from build123d import *

# Parameters (mm, degrees)
SKETCH1_W           = 270
SKETCH1_H           = 180
BOSS_EXTRUDE1_DEPTH = 6
SKETCH2_R           = 1.6
CUT_EXTRUDE1_DEPTH  = 7
SKETCH3_R           = 1.6
CUT_EXTRUDE2_DEPTH  = 10
SKETCH4_R           = 1.6
SKETCH4_R_2         = 1.5
CUT_EXTRUDE3_DEPTH  = 7
SKETCH5_R           = 1.6
CUT_EXTRUDE4_DEPTH  = 10
SKETCH6_R           = 2.1
CUT_EXTRUDE5_DEPTH  = 10


with BuildPart() as part:
    # Sketch1 → Boss-Extrude1 (new body)
    with BuildSketch(Plane(origin=(0, 0, 0), x_dir=(1, 0, 0), z_dir=(0, 1, 0))):
        Rectangle(SKETCH1_W, SKETCH1_H)
    extrude(amount=BOSS_EXTRUDE1_DEPTH)

    # Sketch2 → Cut-Extrude1 (cut, through all)
    with BuildSketch(Plane.XZ):
        with Locations((-122, 81.5)):
            Circle(SKETCH2_R)
        with Locations((-100.000000181, 81.5)):
            Circle(SKETCH2_R)
        with Locations((-122, 6.500000003)):
            Circle(SKETCH2_R)
        with Locations((-100.000000181, 6.500000003)):
            Circle(SKETCH2_R)
        with Locations((-122, 21.000003407)):
            Circle(SKETCH2_R)
        with Locations((-122, 49.000003407)):
            Circle(SKETCH2_R)
    extrude(amount=-CUT_EXTRUDE1_DEPTH, mode=Mode.SUBTRACT)

    # Sketch3 → Cut-Extrude2 (cut)
    with BuildSketch(Plane.XZ):
        with Locations((-40, -39)):
            Circle(SKETCH3_R)
        with Locations((-40, -75)):
            Circle(SKETCH3_R)
        with Locations((-4, -75)):
            Circle(SKETCH3_R)
        with Locations((-4, -39)):
            Circle(SKETCH3_R)
        with BuildLine():
            Line((-29.38, -15.458502607), (-29.38, -5.458502607))
            ThreePointArc((-29.38, -5.458502607), (-27.38, -3.458502607), (-25.38, -5.458502607))
            Line((-25.38, -5.458502607), (-25.38, -15.458502607))
            ThreePointArc((-25.38, -15.458502607), (-27.38, -17.458502607), (-29.38, -15.458502607))
        make_face()
        with BuildLine():
            Line((-14.63, -15.458502607), (-14.63, -5.458502607))
            ThreePointArc((-14.63, -5.458502607), (-16.63, -3.458502607), (-18.63, -5.458502607))
            Line((-18.63, -5.458502607), (-18.63, -15.458502607))
            ThreePointArc((-18.63, -15.458502607), (-16.63, -17.458502607), (-14.63, -15.458502607))
        make_face()
        with BuildLine():
            Line((-29.38, 24.541497393), (-29.38, 34.541497393))
            ThreePointArc((-29.38, 34.541497393), (-27.38, 36.541497393), (-25.38, 34.541497393))
            Line((-25.38, 34.541497393), (-25.38, 24.541497393))
            ThreePointArc((-25.38, 24.541497393), (-27.38, 22.541497393), (-29.38, 24.541497393))
        make_face()
        with BuildLine():
            Line((-14.63, 24.541497393), (-14.63, 34.541497393))
            ThreePointArc((-14.63, 34.541497393), (-16.63, 36.541497393), (-18.63, 34.541497393))
            Line((-18.63, 34.541497393), (-18.63, 24.541497393))
            ThreePointArc((-18.63, 24.541497393), (-16.63, 22.541497393), (-14.63, 24.541497393))
        make_face()
    extrude(amount=-CUT_EXTRUDE2_DEPTH, mode=Mode.SUBTRACT)

    # Sketch4 → Cut-Extrude3 (cut, through all)
    with BuildSketch(Plane(origin=(0, 6, 0), x_dir=(1, 0, 0), z_dir=(0, 1, 0))):
        with Locations((19.999964, -14)):
            Circle(SKETCH4_R)
        with Locations((55.999928, -14.000072)):
            Circle(SKETCH4_R)
        with Locations((20, -50)):
            Circle(SKETCH4_R)
        with Locations((55.999928, -50)):
            Circle(SKETCH4_R)
        with Locations((6.904969305, -32.000108)):
            Circle(SKETCH4_R_2)
        with Locations((6.904969305, -38.817254)):
            Circle(SKETCH4_R_2)
    extrude(amount=-CUT_EXTRUDE3_DEPTH, mode=Mode.SUBTRACT)

    # Sketch5 → Cut-Extrude4 (cut)
    with BuildSketch(Plane(origin=(0, 6, 0), x_dir=(1, 0, 0), z_dir=(0, 1, 0))):
        with Locations((116.5, 10.91154574)):
            Circle(SKETCH5_R)
        with Locations((63.5, 10.91154574)):
            Circle(SKETCH5_R)
        with Locations((116.5, 39.629776512)):
            Circle(SKETCH5_R)
        with Locations((63.5, 39.629776512)):
            Circle(SKETCH5_R)
        with Locations((116.5, 52.91154574)):
            Circle(SKETCH5_R)
        with Locations((63.5, 52.91154574)):
            Circle(SKETCH5_R)
        with Locations((116.5, 81.629776512)):
            Circle(SKETCH5_R)
        with Locations((63.5, 81.629776512)):
            Circle(SKETCH5_R)
        with Locations((125, 76.00062614)):
            Circle(SKETCH5_R)
        with Locations((130, 76.00062614)):
            Circle(SKETCH5_R)
        with Locations((125, 61.00062614)):
            Circle(SKETCH5_R)
        with Locations((130, 61.00062614)):
            Circle(SKETCH5_R)
        with Locations((125, 46.00062614)):
            Circle(SKETCH5_R)
        with Locations((130, 46.00062614)):
            Circle(SKETCH5_R)
        with Locations((125, 31.00062614)):
            Circle(SKETCH5_R)
        with Locations((130, 31.00062614)):
            Circle(SKETCH5_R)
        with Locations((125, 16.00062614)):
            Circle(SKETCH5_R)
        with Locations((130, 16.00062614)):
            Circle(SKETCH5_R)
        with Locations((125, 1.00062614)):
            Circle(SKETCH5_R)
        with Locations((130, 1.00062614)):
            Circle(SKETCH5_R)
        with Locations((125, -13.99937386)):
            Circle(SKETCH5_R)
        with Locations((130, -13.99937386)):
            Circle(SKETCH5_R)
        with Locations((125, -28.99937386)):
            Circle(SKETCH5_R)
        with Locations((130, -28.99937386)):
            Circle(SKETCH5_R)
        with Locations((125, -43.99937386)):
            Circle(SKETCH5_R)
        with Locations((130, -43.99937386)):
            Circle(SKETCH5_R)
    extrude(amount=-CUT_EXTRUDE4_DEPTH, mode=Mode.SUBTRACT)

    # Sketch6 → Cut-Extrude5 (cut)
    with BuildSketch(Plane(origin=(0, 6, 0), x_dir=(1, 0, 0), z_dir=(0, 1, 0))):
        with Locations((15.26, 73)):
            Circle(SKETCH6_R)
        with Locations((43.5, 73)):
            Circle(SKETCH6_R)
        with Locations((15.26, 48)):
            Circle(SKETCH6_R)
        with Locations((43.5, 48)):
            Circle(SKETCH6_R)
        with Locations((15.26, 23)):
            Circle(SKETCH6_R)
        with Locations((43.5, 23)):
            Circle(SKETCH6_R)
    extrude(amount=-CUT_EXTRUDE5_DEPTH, mode=Mode.SUBTRACT)


solid = part.part
Source: CAD feature listing. Evaluate the final solid. Frame: model axes, mm. A direction names the side the tool comes from. Round coordinates to 2 decimals unless told otherwise and drop trailing zeros. Return JSON: item names as keys, results as strings. Group by question number.
1. Reachability of faces 5 (the face through (-18.63, 3, -10)), 6 (the face through (135, 3, 1)) from +Z, -Z, +X, -X, +Y, -Y: full face, straight path, thin tool, end or side. Return the list, or none.
2. Mould query, pull axis Z, two halves, no side actions, for faces 1 (the face through (-2, 3, 90)), 2 (the face through (-18.63, 3, 30)), 3 (the face through (-2, 3, -90)), 4 (the face through (-2, 0, -1)). Classes: released by +Z, released by -Z, zero draft, split by the parting line, or undercut.
3. Pin query (flat end, axial travel): pin 1 (3.5 mm diameter, centred on x = 116.5, z = -39.63, fed in from -Y); pin 2 (2.5 mm diameter, centred on x = 15.26, z = -23, fed in from -Y). Return the tip coordinate at first contact, or that it passes through.
4. Material intervals for line 1 along X through (y, z) = (4.15, -72.5); line 2 along X through (y, z) = (2.4, -23); line 3 along Z through (x, y) = (15.26, 2.7), sorted ascending. Write a range as from..to.
Checks:
{
 "1": {"face 5": "+Y, -Y", "face 6": "+Z, -Z, +X, +Y, -Y"},
 "2": {"face 1": "released by +Z", "face 2": "undercut", "face 3": "released by -Z", "face 4": "zero draft"},
 "3": {"pin 1": "stops at y = 0", "pin 2": "passes through"},
 "4": {"line 1": "x = -135..13.22, 17.3..41.46, 45.54..135", "line 2": "x = -135..13.16, 17.36..41.4, 45.6..135", "line 3": "z = -90..-75.1, -70.9..-50.1, -45.9..-25.1, -20.9..90"}
}
